Input: part model. Units: mm. Frame: model coordinates. Face numbers are marked on the shaded views. A direction names the side the tool comes from. Give positions to 0.01 mm unless a question says otherwise; leave off trailing zeros. Loops run counter-clockwise (first coordinate to the right, second up) from the corner with the lowest first, then second, coordinate; pieces in that order, holes last. Notation, with made-up numbers: (-20.5, 2) - (30.5, 2) arc R3 ccw to (30.5, 6) - close; hole circle Ø3 at (-20.75, 80.25). An arc over 180 degrees is marked (long way). Answer as a JSON object with one key per item and string values. Group by question number.
(1) Section query D-D (y = 61). Return loops of the section in (x, z), plus the area to 3 significant figures.
(2) Material intervals for L1, parallel to X at y = 42, z = 49.5; L2, parallel to X at y = 12, z = 50; L3, parallel to Y at x = 213, z = 78, sorted ascending.
(3) Pin query (flat end, axial travel): P1, Ø10, axis at x = 59, z = 59.5, coming from the +Y side; P2, Ø4, axis at y = 55.5, z = 75.5, coming from the +X side; P3, Ø10, axis at x = 199.5, z = 30, coming from the +Y side. Return the tip coordinate at first contact, or that it passes through.
(4) Section query C-C (y = 45). Return loops of the section in (x, z), plus the area to 3 significant figures.
(5) Mould query, pull axis Z, two halves, no side actions, for the marked faces 1, 2 and 3. Classes: +Z half, -Z half, draft (parallel to the pull), parting line (faces both ways), or undercut.
(6) Section query A-A (z = 55). Return loops of the section in (x, y).
(7) Section query B-B (x = 173). Return loops of the section in (y, z).
(8) Access query for the marked faces 4 and 5. Directions: +Z, -Z, +X, -X, +Y, -Y. A direction counts if a zero-diameter tool reaches every point of the face in a straight line with its end or side. Return the directions, or none.
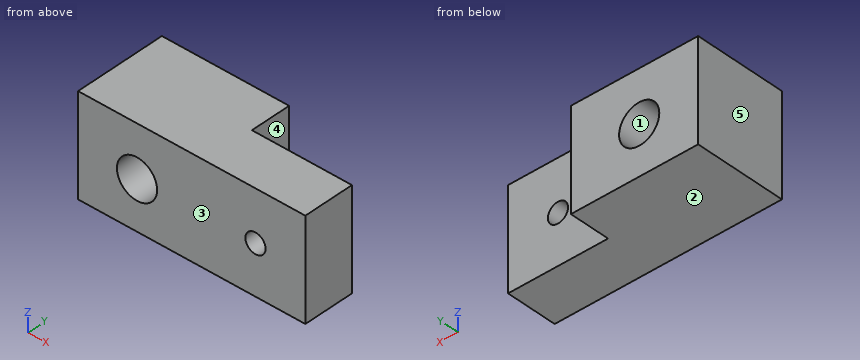
```python
from build123d import *

# Parameters (mm, degrees)
SKETCH1_W             = 127.235427394
SKETCH1_H             = 91.719523319
BOSS_EXTRUDE1_DEPTH   = 100
SKETCH2_W             = 100
SKETCH2_H             = 50.996346368
BOSS_EXTRUDE2_DEPTH   = 100
F_1_0MM_DOWEL_HOLE1_D = 20.2
F_1_0MM_DOWEL_HOLE2_D = 40.2


with BuildPart() as part:
    # Sketch1 → Boss-Extrude1 (new body)
    with BuildSketch(Plane.XY):
        with Locations((63.617713697, 45.85976166)):
            Rectangle(SKETCH1_W, SKETCH1_H)
    extrude(amount=BOSS_EXTRUDE1_DEPTH)

    # Sketch2 → Boss-Extrude2 (add)
    with BuildSketch(Plane(origin=(127.235427394, 0, 0), x_dir=(0, 0, -1), z_dir=(1, 0, 0))):
        with Locations((-50, 25.498173184)):
            Rectangle(SKETCH2_W, SKETCH2_H)
    extrude(amount=BOSS_EXTRUDE2_DEPTH)

    # Ø1.0mm Dowel Hole1 (through all)
    with Locations(Plane(origin=(0, 50.996346368, 0), x_dir=(1, 0, 0), z_dir=(0, 1, 0))):
        with Locations((177.374375047, -49.243565035)):
            Hole(F_1_0MM_DOWEL_HOLE1_D / 2)

    # Ø1.0mm Dowel Hole2 (through all)
    with Locations(Plane(origin=(0, 91.719523319, 0), x_dir=(1, 0, 0), z_dir=(0, 1, 0))):
        with Locations((58.93827193, -48.595192208)):
            Hole(F_1_0MM_DOWEL_HOLE2_D / 2)


solid = part.part
```
Recorded:
{
 "1": {"outline": "(0, 0) - (127.24, 0) - (127.24, 100) - (0, 100) - close; hole circle Ø40.2 at (58.94, 48.6)", "area": "11,500 mm^2"},
 "2": {"L1": "x = 0 to 38.86, 79.02 to 167.28, 187.47 to 227.24", "L2": "x = 0 to 38.89, 78.99 to 167.3, 187.45 to 227.24", "L3": "y = 0 to 51"},
 "3": {"P1": "passes through", "P2": "stops at x = 127.24", "P3": "stops at y = 51"},
 "4": {"outline": "(0, 0) - (227.24, 0) - (227.24, 100) - (0, 100) - close; hole circle Ø40.2 at (58.94, 48.6); hole circle Ø20.2 at (177.37, 49.24)", "area": "21,100 mm^2"},
 "5": {"face 1": "undercut", "face 2": "-Z half", "face 3": "draft"},
 "6": {"outline": "(0, 0) - (39.89, 0) - (39.89, 91.72) - (0, 91.72) - close; (77.99, 0) - (169.08, 0) - (169.08, 51) - (127.24, 51) - (127.24, 91.72) - (77.99, 91.72) - close; (185.67, 0) - (227.24, 0) - (227.24, 51) - (185.67, 51) - close"},
 "7": {"outline": "(0, 0) - (51, 0) - (51, 40.14) - (0, 40.14) - close; (0, 58.35) - (51, 58.35) - (51, 100) - (0, 100) - close"},
 "8": {"face 4": "+Z, -Z, +X, +Y", "face 5": "+Z, -Z, -X, +Y, -Y"}
}
